Part model, mm, in its own coordinate system. Face numbers are marked on the shaded views. Round coordinates to 2 decimals unless told otherwise and drop trailing zeros. Loops run counter-clockwise (first coordinate to the right, second up) from the corner with the lowest first, then second, coordinate; pieces in that order, holes last. Notation, with made-up numbers: M -32,79.5 L 26,79.5 A14 cw 26,95.5 Z; hole C 14,44.5 d6. An arc over 180 degrees is marked long. Put each result on its own line as item: value. Start each with the question number.
1) Slice it at B-B on y = 4. Give the cut face in (x, z).
2) Probe line 1 along X through (y, z) = (-13, -1.4); line 2 along Y through (x, z) = (-3, -2.25). List the from-to ranges inside material, lowest first.
3) Slice it at A-A on z = -1.65. State how many separate pieces and enclosed holes the cut face has, then the cut area to 3 significant figures.
4) Pull direction Y, two halves, no side cores. Call the marked faces 1, 2, 3 and 4: +Y half, -Y half, draft (parallel to the pull), parting line (faces both ways), or undercut.
5) Drop a flat-ended pin along its axis: pin 1 Ø2.5 at (x, y) = (-1, -0.5) entering from -Z. Give the stop position or say it passes through.
```python
from build123d import *

# Parameters (mm, degrees)
SKETCH021_W                      = 31.8
SKETCH021_H                      = 31.8
PAD014_DEPTH                     = 3.05
SKETCH022_W                      = 28.8
SKETCH022_H                      = 28.8
POCKET008_DEPTH                  = 2.2
SKETCH023_R                      = 3.25
SKETCH023_R_2                    = 2.45
PAD015_DEPTH                     = 2.2
SKETCH023_LINEARPATTERN002_2_R   = 3.25
SKETCH023_LINEARPATTERN002_2_R_2 = 2.45
PAD015_LINEARPATTERN002_2_DEPTH  = 2.2
SKETCH023_LINEARPATTERN002_3_R   = 3.25
SKETCH023_LINEARPATTERN002_3_R_2 = 2.45
PAD015_LINEARPATTERN002_3_DEPTH  = 2.2
LINEARPATTERN003_COUNT           = 3
LINEARPATTERN003_PITCH           = 8
BODY005_PLACEMENT_ANGLE          = 180


with BuildPart() as part:
    # Sketch021 → Pad014 (new body)
    with BuildSketch(Plane.XY):
        Rectangle(SKETCH021_W, SKETCH021_H)
    extrude(amount=PAD014_DEPTH)

    # Sketch022 (on Face6 of Pad014) → Pocket008 (cut)
    with BuildSketch(Plane.XY.offset(3.05)):
        Rectangle(SKETCH022_W, SKETCH022_H)
    extrude(amount=-POCKET008_DEPTH, mode=Mode.SUBTRACT)

    # Sketch023 (on Face11 of Pocket008) → Pad015 (join)
    with BuildSketch(Plane.XY.offset(0.85)):
        with Locations((8, 8)):
            Circle(SKETCH023_R)
        with Locations((8, 8)):
            Circle(SKETCH023_R_2, mode=Mode.SUBTRACT)
    pad015 = extrude(amount=PAD015_DEPTH)

    # Sketch023 LinearPattern002 2 → Pad015 LinearPattern002 2 (add)
    with BuildSketch(Plane(origin=(-8, 0, 0.85), x_dir=(1, 0, 0), z_dir=(0, 0, 1))):
        with Locations((8, 8)):
            Circle(SKETCH023_LINEARPATTERN002_2_R)
        with Locations((8, 8)):
            Circle(SKETCH023_LINEARPATTERN002_2_R_2, mode=Mode.SUBTRACT)
    pad015_linearpattern002_2 = extrude(amount=PAD015_LINEARPATTERN002_2_DEPTH)

    # Sketch023 LinearPattern002 3 → Pad015 LinearPattern002 3 (add)
    with BuildSketch(Plane(origin=(-16, 0, 0.85), x_dir=(1, 0, 0), z_dir=(0, 0, 1))):
        with Locations((8, 8)):
            Circle(SKETCH023_LINEARPATTERN002_3_R)
        with Locations((8, 8)):
            Circle(SKETCH023_LINEARPATTERN002_3_R_2, mode=Mode.SUBTRACT)
    pad015_linearpattern002_3 = extrude(amount=PAD015_LINEARPATTERN002_3_DEPTH)

    # LinearPattern003: Pad015, Pad015 LinearPattern002 2, Pad015 LinearPattern002 3 ×3
    with Locations(*[(0, -i * LINEARPATTERN003_PITCH, 0) for i in range(1, LINEARPATTERN003_COUNT)]):
        add(pad015)
        add(pad015_linearpattern002_2)
        add(pad015_linearpattern002_3)


with BuildPart() as part_1:
    # Body005 placement: moved
    add(part.part.moved(Location((0, 0, -0.15))).rotate(Axis((0, 0, -0.15), (0, 1, 0)), BODY005_PLACEMENT_ANGLE))


solid = part_1.part
```
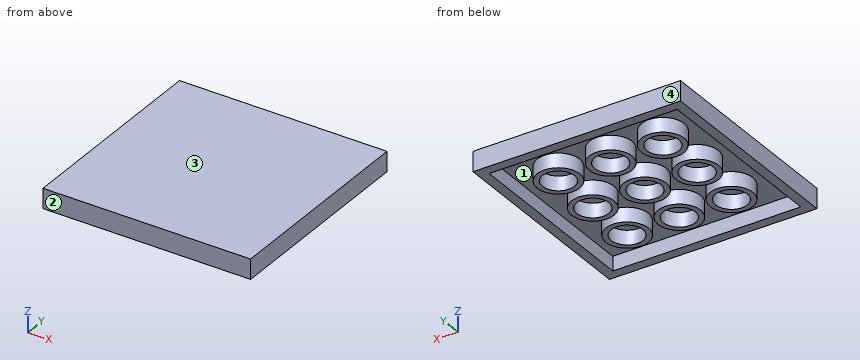
Recorded:
1. outline: M -15.9,-3.2 L -14.4,-3.2 L -14.4,-1 L 14.4,-1 L 14.4,-3.2 L 15.9,-3.2 L 15.9,-0.15 L -15.9,-0.15 Z
2. line 1: x = -15.9 to -14.4, 14.4 to 15.9
2. line 2: y = -15.9 to -14.4, -9.25 to -6.75, -1.25 to 1.25, 6.75 to 9.25, 14.4 to 15.9
3. separate pieces: 10
3. enclosed holes: 10
3. area: 311 mm2
4. face 1: undercut
4. face 2: -Y half
4. face 3: draft
4. face 4: +Y half
5. pin 1: stops at z = -1
